Check sheet for the modelled part. Datum: model origin and axes. Units: mm. Face numbers are marked on the shaded views. A direction names the side the tool comes from. Round coordinates to 2 decimals unless told otherwise and drop trailing zeros. Order: outer loops, then holes, each group sorted by start corner. A loop starts at its lowest first (then second) coordinate and runs counter-clockwise, first axis right, second up. Notation, with made-up numbers: (-21.75, 19.5) -> (13.25, 19.5) arc R23 ccw to (13.25, 38.5) -> close; hole circle Ø4 at (36, 48.25). An arc over 180 degrees is marked (long way). Answer in a Markdown table with one row per item.
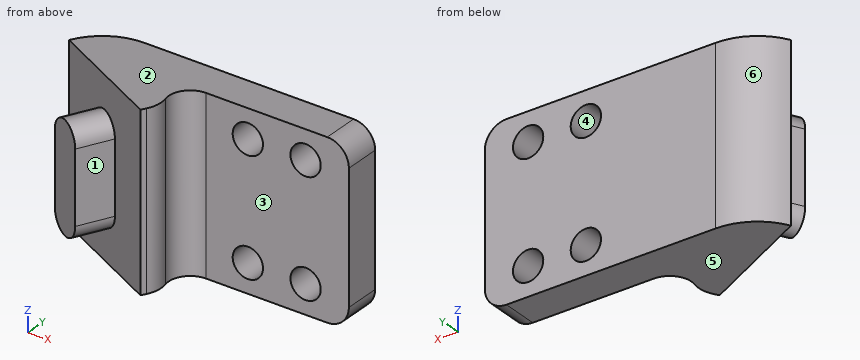
```python
from build123d import *

# Parameters (mm, degrees)
ESQUISSE1_W             = 17
ESQUISSE1_H             = 5
BOSS_EXTRU_1_DEPTH      = 24
BOSS_EXTRU_2_DEPTH      = 24
CONG_1_R                = 4
CONG_2_R                = 8
CONG_3_R                = 3
ESQUISSE3_W             = 24
ESQUISSE3_H             = 5
BOSS_EXTRU_3_DEPTH      = 10
ESQUISSE4_R             = 2.1
ENL_V_MAT_EXTRU_1_DEPTH = 10
CONG_4_R                = 3
BOSS_EXTRU_4_DEPTH      = 5


with BuildPart() as part:
    # Esquisse1 → Boss.-Extru.1 (new body)
    with BuildSketch(Plane.XY):
        with Locations((1.940369129, 2.5)):
            Rectangle(ESQUISSE1_W, ESQUISSE1_H)
    extrude(amount=BOSS_EXTRU_1_DEPTH)

    # Esquisse2 → Boss.-Extru.2 (add)
    with BuildSketch(Plane.XY.offset(24)):
        Polygon((-18.723069156, 0.535871193), (-3.080508445, -7.355303518), (-0.501566554, -3.056100904), (-16.471058056, 5), align=None)
        Polygon((-6.559630871, 0), (-6.559630871, 5), (-16.471058056, 5), align=None)
    extrude(amount=-BOSS_EXTRU_2_DEPTH)

    # Congé1
    cong_1_edges = [part.edges().sort_by_distance(p)[0] for p in [
        (-0.501566554, -3.056100904, 12),
    ]]
    fillet(cong_1_edges, radius=CONG_1_R)

    # Congé2
    cong_2_edges = [part.edges().sort_by_distance(p)[0] for p in [
        (-16.471058056, 5, 12),
    ]]
    fillet(cong_2_edges, radius=CONG_2_R)

    # Congé3
    cong_3_edges = [part.edges().sort_by_distance(p)[0] for p in [
        (-6.559630871, 0, 12),
    ]]
    fillet(cong_3_edges, radius=CONG_3_R)

    # Esquisse3 → Boss.-Extru.3 (add)
    with BuildSketch(Plane(origin=(10.440369129, 0, 0), x_dir=(0, 0, -1), z_dir=(1, 0, 0))):
        with Locations((-12, 2.5)):
            Rectangle(ESQUISSE3_W, ESQUISSE3_H)
    extrude(amount=BOSS_EXTRU_3_DEPTH)

    # Esquisse4 → Enlèv. mat.-Extru.1 (cut)
    with BuildSketch(Plane(origin=(0, 5, 0), x_dir=(1, 0, 0), z_dir=(0, 1, 0))):
        with Locations(Location((6.440369129, -20, 0), (0, 0, 270))):
            Circle(ESQUISSE4_R)
        with Locations(Location((14.440369129, -20, 0), (0, 0, 270))):
            Circle(ESQUISSE4_R)
        with Locations(Location((14.440369129, -4, 0), (0, 0, 270))):
            Circle(ESQUISSE4_R)
        with Locations(Location((6.440369129, -4, 0), (0, 0, 270))):
            Circle(ESQUISSE4_R)
    extrude(amount=-ENL_V_MAT_EXTRU_1_DEPTH, mode=Mode.SUBTRACT)

    # Congé4
    cong_4_edges = [part.edges().sort_by_distance(p)[0] for p in [
        (20.440369129, 2.5, 0),
        (20.440369129, 2.5, 24),
    ]]
    fillet(cong_4_edges, radius=CONG_4_R)

    # Esquisse5 → Boss.-Extru.4 (add)
    with BuildSketch(Plane(origin=(-3.582711985, -7.101957793, 0), x_dir=(0.892825761431464, -0.45040221993716517, 0), z_dir=(-0.45040221993716517, -0.892825761431464, 0))):
        with BuildLine():
            Line((-5.697654158, 17), (-5.697654158, 7))
            ThreePointArc((-5.697654158, 7), (-8.197654158, 4.5), (-10.697654158, 7))
            Line((-10.697654158, 7), (-10.697654158, 17))
            ThreePointArc((-10.697654158, 17), (-8.197654158, 19.5), (-5.697654158, 17))
        make_face()
    extrude(amount=BOSS_EXTRU_4_DEPTH)


solid = part.part
```
(1) Section check A-A on y = 2.25. Record the boundary of the cut face in (x, z).
Solutions:
| item | result |
|---|---|
| outline | (-17.58, 0) -> (17.44, 0) arc R3 ccw to (20.44, 3) -> (20.44, 21) arc R3 ccw to (17.44, 24) -> (-17.58, 24) -> close; hole circle Ø4.2 at (6.44, 4); hole circle Ø4.2 at (6.44, 20); hole circle Ø4.2 at (14.44, 4); hole circle Ø4.2 at (14.44, 20) |
(2) Scan lines: probe 1 along X at (y, z) = (1.85, 20); probe 2 along Z at (x, y) = (8, 3); probe 3 along Y at (x, z) = (6.5, 6.25). Record each from-to range of solid material in increasing order. Write a range as from..to.
Solutions:
| item | result |
|---|---|
| probe 1 | -17.91..4.34, 8.54..12.34, 16.54..20.44 |
| probe 2 | 0..2.59, 5.41..18.59, 21.41..24 |
| probe 3 | 0..5 |
(3) Draft check along X on the marked faces 4, 5 and 6. Enter one of: pulls with the +X half, pulls with the -X half, needs draft (parallel to the pull), parting line crosses it, or undercut.
Solutions:
| item | result |
|---|---|
| face 4 | undercut |
| face 5 | needs draft |
| face 6 | pulls with the -X half |
(4) Tool access check on the marked faces 1, 2 and 3. Record the directions out of +Z, -Z, +X, -X, +Y, -Y that give a thin tool (end or side, any length) a straight path to the whole face; none if there is none.
Solutions:
| item | result |
|---|---|
| face 1 | +Z, -Z, -Y |
| face 2 | +Z, +X, -X, +Y, -Y |
| face 3 | +Z, -Z, +X, -Y |
(5) Section check B-B on z = 4. Give the number of separate pieces and of enclosed holes in the cut face, plus the area to 3 significant figures.
Solutions:
| item | result |
|---|---|
| separate pieces | 3 |
| enclosed holes | 0 |
| area | 205 mm^2 |
(6) Depth check by flat-ended pin: pin 1 Ø8 at (x, y) = (-14, -6.5) entering from -Z; pin 2 Ø5 at (x, z) = (14.44, 4) entering from -Y; pin 3 Ø2 at (y, z) = (-6, 7) entering from +X. Enter the tip coordinate at first touch or a pass-through.
Solutions:
| item | result |
|---|---|
| pin 1 | z = 4.5 |
| pin 2 | y = 0 |
| pin 3 | x = -2.16 |
